Geometry check sheet. Reference: the model listing, model coordinates, mm. Give positions to 0.01 mm unless a question says otherwise; leave off trailing zeros. Loops run counter-clockwise (first coordinate to the right, second up) from the corner with the lowest first, then second, coordinate; pieces in that order, holes last.
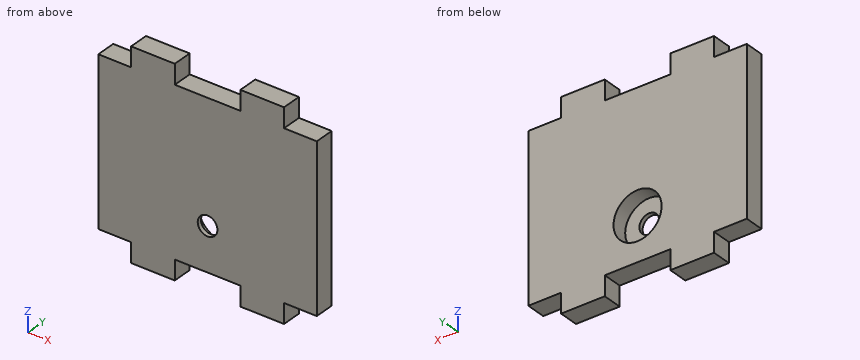
```python
from build123d import *

# Parameters (mm, degrees)
BOSS_EXTRUDE1_DEPTH = 9
SKETCH3_R           = 11
CUT_EXTRUDE1_DEPTH  = 7.05


with BuildPart() as part:
    # Sketch2 → Boss-Extrude1 (new body)
    with BuildSketch(Plane(origin=(0, 0, 0), x_dir=(1, 0, 0), z_dir=(0, 1, 0))):
        Polygon((-35, 37.5), (-50, 37.5), (-50, -37.5), (-35, -37.5), (-35, -46.5), (-15, -46.5), (-15, -37.5), (15, -37.5), (15, -46.5), (35, -46.5), (35, -37.5), (50, -37.5), (50, 37.5), (35, 37.5), (35, 46.5), (15, 46.5), (15, 37.5), (-15, 37.5), (-15, 46.5), (-35, 46.5), align=None)
        with BuildLine():
            ThreePointArc((4.5, 17.5), (0, 13), (-4.5, 17.5))
            ThreePointArc((-4.5, 17.5), (0, 22), (4.5, 17.5))
        make_face(mode=Mode.SUBTRACT)
    extrude(amount=BOSS_EXTRUDE1_DEPTH)

    # Sketch3 → Cut-Extrude1 (cut)
    with BuildSketch(Plane(origin=(0, 9, 0), x_dir=(1, 0, 0), z_dir=(0, 1, 0))):
        with Locations(Location((0, 17.5, 0), (0, 0, 270))):
            Circle(SKETCH3_R)
    extrude(amount=-CUT_EXTRUDE1_DEPTH, mode=Mode.SUBTRACT)


solid = part.part
```
1) Sectioned sample at C-C on x = 0. Enter the section's corners in (y, z).
2) Depth check by flat-ended pin: P1, Ø6.5, axis at x = 0, z = -16.5, coming from the +Y side; P2, Ø10.5, axis at x = 0, z = -17.5, coming from the -Y side; P3, Ø2.5, axis at y = 6.5, z = -41.5, coming from the +X side; P4, Ø1.5, axis at x = -4, y = 4, coming from the -Z side. Enter the tip coordinate at first touch or a pass-through.
3) Sectioned sample at B-B on y = 4. Enter the section's corners in (x, z), plus the area to 3 significant figures.
4) Sectioned sample at A-A on z = -17.5. Enter the section's corners in (x, y).
5) Sectioned sample at D-D on x = 41.5. Enter the section's corners in (y, z), plus the area to 3 significant figures.
6) Scan lines: line 1 along Z through (x, y) = (0, 1.2); line 2 along X through (y, z) = (1.45, -17.5); line 3 along X through (y, z) = (4, -17.5). Record each from-to range of solid material in increasing order.
Determined:
1. outline: (0, -37.5) - (9, -37.5) - (9, -28.5) - (1.95, -28.5) - (1.95, -22) - (0, -22) - close; (0, -13) - (1.95, -13) - (1.95, -6.5) - (9, -6.5) - (9, 37.5) - (0, 37.5) - close
2. P1: passes through
2. P2: stops at y = 0
2. P3: stops at x = 35
2. P4: stops at z = -37.5
3. outline: (-50, -37.5) - (-35, -37.5) - (-35, -46.5) - (-15, -46.5) - (-15, -37.5) - (15, -37.5) - (15, -46.5) - (35, -46.5) - (35, -37.5) - (50, -37.5) - (50, 37.5) - (35, 37.5) - (35, 46.5) - (15, 46.5) - (15, 37.5) - (-15, 37.5) - (-15, 46.5) - (-35, 46.5) - (-35, 37.5) - (-50, 37.5) - close; hole circle Ø22 at (0, -17.5)
3. area: 7,840 mm2
4. outline: (-50, 0) - (-4.5, 0) - (-4.5, 1.95) - (-11, 1.95) - (-11, 9) - (-50, 9) - close; (4.5, 0) - (50, 0) - (50, 9) - (11, 9) - (11, 1.95) - (4.5, 1.95) - close
5. outline: (0, -37.5) - (9, -37.5) - (9, 37.5) - (0, 37.5) - close
5. area: 675 mm2
6. line 1: z = -37.5 to -22, -13 to 37.5
6. line 2: x = -50 to -4.5, 4.5 to 50
6. line 3: x = -50 to -11, 11 to 50
